Could you check a few things on this drawing? It's one solid part, dimensions in mm from its lowest x, y, z. A direction names the side the tool comes from. Round coordinates to 2 decimals unless told otherwise and drop trailing zeros. Order: outer loops, then holes, each group sorted by start corner. A loop starts at its lowest first (then second) coordinate and runs counter-clockwise, first axis right, second up. Notation, with made-up numbers: (-31, 63) -> (23, 63) arc R15 ccw to (23, 76) -> close; hole circle Ø3 at (4.5, 46.25). An arc over 180 degrees is marked (long way). Use a Markdown table: item, result. Add a question column.
(1) If I drill on probe 1 along Z at (x, y) = (266.7, 2.5) (3 decimals); probe 2 along Z at (x, y) = (266, 2); probe 3 along Y at (x, z) = (29.5, 50.5), over which ranges is the centre line in solid material (lowest first)?
(2) On a 3-axis mill with a long thin cutter (end or side, diameter ignored), from which of +Z, -Z, +X, -X, +Y, -Y can I reach the whole of each face in a straight line? I mean the marked faces 4, 5 and 6. Say none if no direction works.
(3) I want a section at B-B, the plane y = 133. Please give me the cut outline in (x, z), then the cut area to 3 significant figures.
(4) I want a section at A-A, the plane z = 42. Please give me the cut outline in (x, y).
(5) Thinking about a two-plate mould opening in X: for the marked faces 1, 2 and 3, which applies, pulls with the +X half, pulls with the -X half, needs draft (parallel to the pull), parting line crosses it, or undercut?
(6) I'm going to push flat-ended pins straight in: P1, Ø7.5, axis at x = 266.7, z = 31.75, coming from the +Y side; P2, Ø8, axis at y = 44.5, z = 47, coming from the +X side; P3, Ø4, axis at y = 122.5, z = 48, coming from the -X side. Where does each tip first touch, or does it pass through?
(7) I want a section at C-C, the plane x = 488. Please give me the cut outline in (y, z).
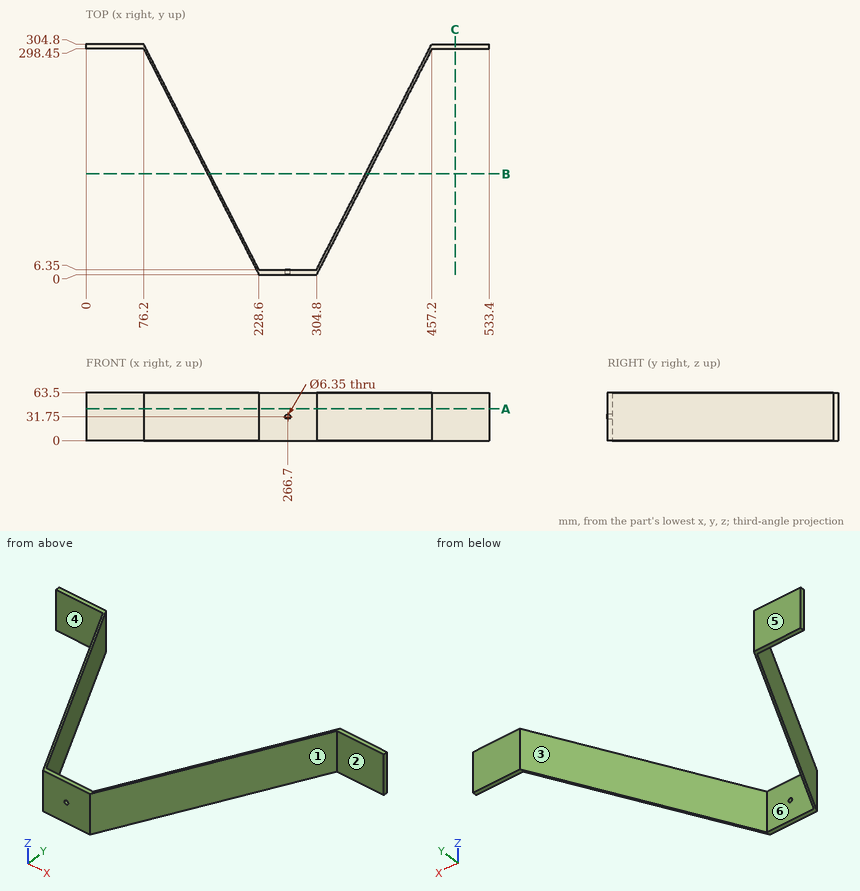
Taken from the geometry:
| question | item | result |
|---|---|---|
| 1 | probe 1 | z = 0 to 28.575, 34.925 to 63.5 |
| 1 | probe 2 | z = 0 to 28.65, 34.85 to 63.5 |
| 1 | probe 3 | y = 298.45 to 304.8 |
| 2 | face 4 | +Z, -Z, -X, -Y |
| 2 | face 5 | +Z, -Z, +X, -X, +Y |
| 2 | face 6 | +Z, -Z, +Y |
| 3 | outline | (160.69, 0) -> (163.93, 0) -> (163.93, 63.5) -> (160.69, 63.5) -> close; (369.47, 0) -> (372.71, 0) -> (372.71, 63.5) -> (369.47, 63.5) -> close |
| 3 | area | 412 mm2 |
| 4 | outline | (0, 298.45) -> (76.2, 298.45) -> (228.6, 0) -> (304.8, 0) -> (457.2, 298.45) -> (533.4, 298.45) -> (533.4, 304.8) -> (457.2, 304.8) -> (304.8, 6.35) -> (228.6, 6.35) -> (76.2, 304.8) -> (0, 304.8) -> close |
| 5 | face 1 | pulls with the +X half |
| 5 | face 2 | needs draft |
| 5 | face 3 | undercut |
| 6 | P1 | stops at y = 6.35 |
| 6 | P2 | stops at x = 329.57 |
| 6 | P3 | stops at x = 165.03 |
| 7 | outline | (298.45, 0) -> (304.8, 0) -> (304.8, 63.5) -> (298.45, 63.5) -> close |
